For this review, take the finished solid that the model builds, in its own axes (mm). A direction names the side the tool comes from. Coordinates: 2 decimals unless noted, no trailing zeros. Write each loop counter-clockwise with the first axis right and the second up, starting at its lowest first coordinate (ties: lowest second). Pieces come first, ordered by that corner, then holes. Notation, with made-up numbers: (3, 34) -> (42, 34) arc R11 ccw to (42, 50) -> close; hole circle Ø10 at (83, -29.75). An arc over 180 degrees is marked (long way). One line per item, written item: value. Start each with the question number.
1) Add section D-D (x = 49). State the section outline as (y, z) points, and give its area (3 significant figures).
2) For pin 1 Ø1.5 at (x, y) = (27.5, 4) entering from +Z; pin 2 Ø6 at (x, y) = (57.5, 6) entering from -Z; pin 3 Ø2.5 at (x, z) = (0, 0) entering from +Y; pin 4 Ø6 at (y, z) = (3.5, 4) entering from -X, all flat-tipped, find the tip position at first contact; note any pin that passes through.
3) Add section A-A (z = 0). State the section outline as (x, y) points, and give its area (3 significant figures).
4) Add section B-B (x = 4). State the section outline as (y, z) points, and give its area (3 significant figures).
5) Machinability: for faces 1 (the flat face through (51, 1, 0)), 2 (the flat face through (51, 5, -5)), 3 (the flat face through (5, 5, 0)), 4 (the flat face through (51, 5, 5)), 5 (the flat face through (90, 5, 0)), which of the approach directions +Z, -Z, +X, -X, +Y, -Y give a long, thin tool a straight path to every point of the face, cutting with its end or side? Answer none if there is none.
6) For probe 1 along X at (y, z) = (1.05, 0); probe 2 along X at (y, z) = (0.7, 0); probe 3 along Y at (x, z) = (-1.5, 3.5), list the stretches that pass through material, from the lowest coordinate up. Write a range as from..to.
7) Add section C-C (y = 5.75). State the section outline as (x, z) points, and give its area (3 significant figures).
8) Mouldability with a two-part tool opening along X and no side actions: class faces 6 (the cylindrical face through (-1.5, 9.24, -0.07)), 7 (the cylindrical face through (-1.5, 0.74, -0.07)), 8 (the cylindrical face through (-6, 1, 0)), 9 (the flat face through (51, 9, 0)) as released by +X, released by -X, zero draft, split by the parting line, or undercut.
from build123d import *

# Parameters (mm, degrees)
SZKIC1_R                    = 1.5
DODANIE_WYCI_GNI_CIE1_DEPTH = 10
SZKIC2_W                    = 22
SZKIC2_H                    = 7
WYTNIJ_WYCI_GNI_CIE1_DEPTH  = 13
SZKIC3_OUTSIDE_W            = 33.452
SZKIC3_OUTSIDE_H            = 31.452
SZKIC3_OUTSIDE_W_2          = 10
SZKIC3_OUTSIDE_H_2          = 8
WYTNIJ_WYCI_GNI_CIE2_DEPTH  = 80


with BuildPart() as part:
    # Szkic1 → Dodanie-wyciągnięcie1 (new body)
    with BuildSketch(Plane(origin=(0, 0, 0), x_dir=(1, 0, 0), z_dir=(0, 1, 0))):
        with BuildLine():
            Line((90, 6), (90, -6))
            Line((90, -6), (0, -6))
            ThreePointArc((0, -6), (-6, 0), (0, 6))
            Line((0, 6), (90, 6))
        make_face()
        Circle(SZKIC1_R, mode=Mode.SUBTRACT)
    extrude(amount=DODANIE_WYCI_GNI_CIE1_DEPTH)

    # Szkic2 → Wytnij-wyciągnięcie1 (cut, through all)
    with BuildSketch(Plane(origin=(0, 0, -6), x_dir=(-1, 0, 0), z_dir=(0, 0, -1))):
        with Locations((6, 5)):
            Rectangle(SZKIC2_W, SZKIC2_H)
    extrude(amount=-WYTNIJ_WYCI_GNI_CIE1_DEPTH, mode=Mode.SUBTRACT)

    # Szkic3 outside → Wytnij-wyciągnięcie2 (cut)
    with BuildSketch(Plane(origin=(90, 0, 0), x_dir=(0, 0, -1), z_dir=(1, 0, 0))):
        with Locations((0, 5)):
            Rectangle(SZKIC3_OUTSIDE_W, SZKIC3_OUTSIDE_H)
        with Locations((0, 5)):
            Rectangle(SZKIC3_OUTSIDE_W_2, SZKIC3_OUTSIDE_H_2, mode=Mode.SUBTRACT)
    extrude(amount=-WYTNIJ_WYCI_GNI_CIE2_DEPTH, mode=Mode.SUBTRACT)


solid = part.part
Numbers:
1. outline: (1, -5) -> (9, -5) -> (9, 5) -> (1, 5) -> close
1. area: 80.0 mm²
2. pin 1: z = 5
2. pin 2: z = -5
2. pin 3: through
2. pin 4: x = -5.73
3. outline: (-6, 0) -> (-1.5, 0) -> (-1.5, 1.5) -> (-6, 1.5) -> close; (-6, 8.5) -> (-1.5, 8.5) -> (-1.5, 10) -> (-6, 10) -> close; (1.5, 0) -> (10, 0) -> (10, 1) -> (90, 1) -> (90, 9) -> (10, 9) -> (10, 10) -> (1.5, 10) -> (1.5, 8.5) -> (5, 8.5) -> (5, 1.5) -> (1.5, 1.5) -> close
3. area: 714 mm²
4. outline: (0, -6) -> (1.5, -6) -> (1.5, 6) -> (0, 6) -> close; (8.5, -6) -> (10, -6) -> (10, 6) -> (8.5, 6) -> close
4. area: 36.0 mm²
5. face 1: +Z, -Z, +X, -Y
5. face 2: -Z, +X, +Y, -Y
5. face 3: +Z, -Z, -X
5. face 4: +Z, +X, +Y, -Y
5. face 5: +Z, -Z, +X, +Y, -Y
6. probe 1: -6..-1.5, 1.5..90
6. probe 2: -6..-1.5, 1.5..10
6. probe 3: 0..1.5, 8.5..10
7. outline: (5, -6) -> (10, -6) -> (10, -5) -> (90, -5) -> (90, 5) -> (10, 5) -> (10, 6) -> (5, 6) -> close
7. area: 860 mm²
8. face 6: undercut
8. face 7: undercut
8. face 8: released by -X
8. face 9: zero draft
